Drawing for the job (mm, zero at the part's lowest x, y, z). A direction names the side the tool comes from. Coordinates: 2 decimals unless noted, no trailing zeros. Order: outer loops, then holes, each group sorted by start corner. A loop starts at its lowest first (then second) coordinate and runs counter-clockwise, first axis right, second up. Notation, with made-up numbers: (51.5, -36.75) - (82.5, -36.75) arc R9 ccw to (82.5, -19.75) - close; hole circle Ø6 at (-5, 82). An arc over 180 degrees is marked (long way). Put each result on its own line as item: value. Start each with the question number.
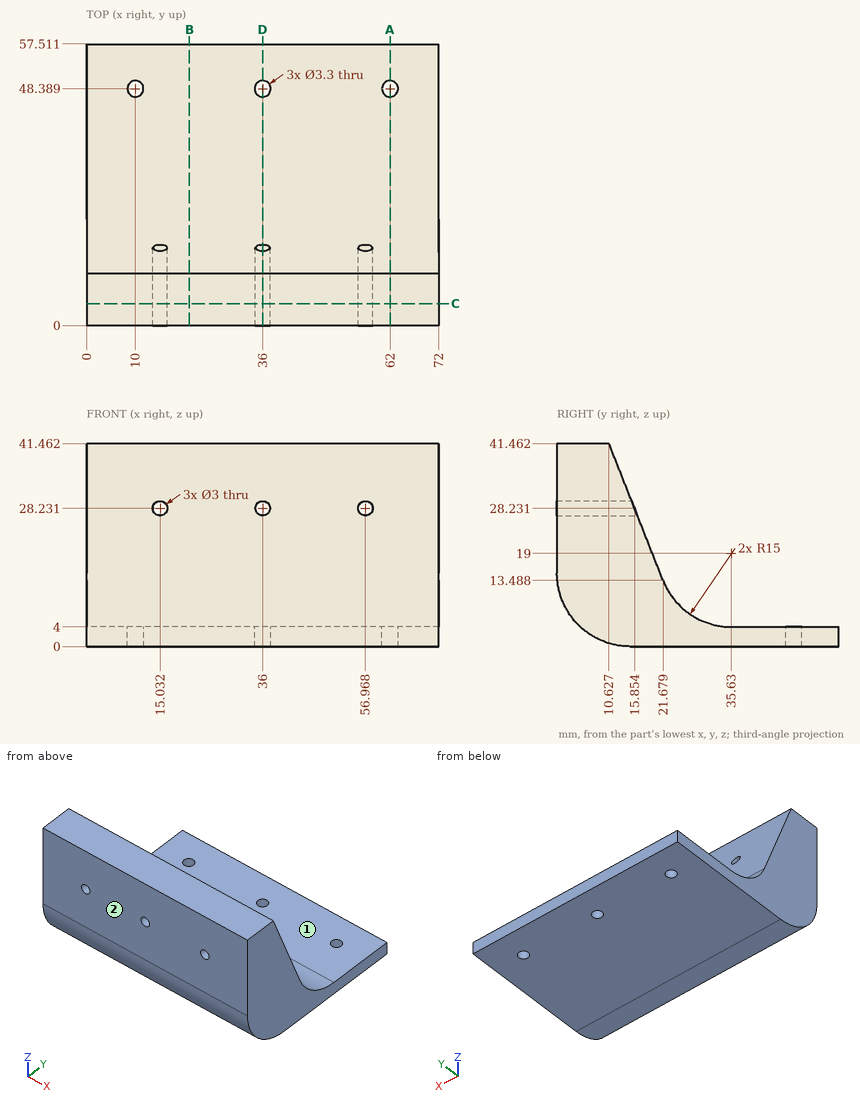
Item 1: Wall check: line 1 along Z through (x, y) = (32, 43); line 2 along Y through (x, z) = (62, 2) (1 decimal); line 3 along X through (y, z) = (9.5, 29) (1 decimal). Give the ranges that are in metal, low to high.
Item 2: Slice it at A-A, the plane x = 62. Give the cut face in (y, z).
Item 3: Flat gauge pins, fed straight in: pin 1 Ø17.5 at (x, y) = (21, 52) entering from +Z; pin 2 Ø1.8 at (x, z) = (56.97, 28.23) entering from -Y; pin 3 Ø2 at (x, z) = (17.5, 14.5) entering from +Y (1 decimal). Where does each tip first touch, or does it go through?
Item 4: Slice it at D-D, the plane x = 36. Give the cut face in (y, z), plus the area to 3 significant figures.
Item 5: Slice it at C-C, the plane y = 4.5. Give the cut face in (x, z).
Item 6: Slice it at B-B, the plane x = 21. Give the cut face in (y, z).
Item 7: 3-axis set-ups, long thin cutter, end or side, ignore diameter. For the marked faces 1 and 2: which of +Z, -Z, +X, -X, +Y, -Y reach the whole face in a straight line?
Here are the results:
1. line 1: z = 0 to 4
1. line 2: y = 7.5 to 46.7, 50 to 57.5
1. line 3: x = 0 to 13.7, 16.3 to 34.7, 37.3 to 55.7, 58.3 to 72
2. outline: (0, 15) arc R15 ccw to (15, 0) - (46.74, 0) - (46.74, 4) - (35.63, 4) arc R15 cw to (21.68, 13.49) - (10.63, 41.46) - (0, 41.46) - close; (50.04, 0) - (57.51, 0) - (57.51, 4) - (50.04, 4) - close
3. pin 1: stops at z = 4
3. pin 2: passes through
3. pin 3: stops at y = 21.7
4. outline: (0, 15) arc R15 ccw to (15, 0) - (46.74, 0) - (46.74, 4) - (35.63, 4) arc R15 cw to (21.68, 13.49) - (16.45, 26.73) - (0, 26.73) - close; (0, 29.73) - (15.26, 29.73) - (10.63, 41.46) - (0, 41.46) - close; (50.04, 0) - (57.51, 0) - (57.51, 4) - (50.04, 4) - close
4. area: 815 mm^2
5. outline: (0, 4.29) - (72, 4.29) - (72, 41.46) - (0, 41.46) - close; hole circle Ø3 at (15.03, 28.23); hole circle Ø3 at (36, 28.23); hole circle Ø3 at (56.97, 28.23)
6. outline: (0, 15) arc R15 ccw to (15, 0) - (57.51, 0) - (57.51, 4) - (35.63, 4) arc R15 cw to (21.68, 13.49) - (10.63, 41.46) - (0, 41.46) - close
7. face 1: +Z, +X, -X, +Y
7. face 2: +Z, -Z, +X, -X, -Y
